```python
from build123d import *

# Parameters (mm, degrees)
EXTRUDE_1_DEPTH              = 5
HOLE_WIZARD_M4_1_D           = 4.3
HOLE_WIZARD_M4_1_CSINK_D     = 8.6
HOLE_WIZARD_M4_1_CSINK_ANGLE = 90
FILLET_1_R                   = 1


with BuildPart() as part:
    # 草图1 → 凸台-拉伸1 (new body)
    with BuildSketch(Plane(origin=(0, 0, 0), x_dir=(0, 0, -1), z_dir=(1, 0, 0))):
        Polygon((22, 18), (15.44969994, 18), (16.349099819, 8), (43.650900181, 8), (44.55030006, 18), (38, 18), align=None)
    extrude(amount=EXTRUDE_1_DEPTH)

    # M4 十字槽沉头木螺钉的锥形沉头孔1 (through all)
    with Locations(Plane.ZY):
        with Locations((-38, 13), (-22, 13)):
            CounterSinkHole(HOLE_WIZARD_M4_1_D / 2, HOLE_WIZARD_M4_1_CSINK_D / 2, counter_sink_angle=HOLE_WIZARD_M4_1_CSINK_ANGLE)

    # 圆角1
    # the kernel refuses this fillet: 1 mm, written as the material it takes off along each edge
    with BuildSketch(Plane(origin=(1, 9, -17.263196285), x_dir=(0, -0.08957840876297431, 0.9959797732301061), z_dir=(-1, 0, 0))) as fillet_1_piece_1_section:
        Polygon((0, 0), (FILLET_1_R, 0), (FILLET_1_R, -FILLET_1_R * 0.914096466321), (FILLET_1_R * 0.089578408763, -FILLET_1_R * 0.99597977323), align=None)
    fillet_1_piece_1 = extrude(amount=FILLET_1_R, mode=Mode.PRIVATE)
    fillet_1_piece_1 = fillet_1_piece_1 - Plane(origin=(1, 9, -17.263196285), x_dir=(0, 0.7380983703961737, -0.6746931121765753), z_dir=(-1, 0, 0)) * Sphere(FILLET_1_R, mode=Mode.PRIVATE)
    add(fillet_1_piece_1, mode=Mode.SUBTRACT)
    with BuildSketch(Plane(origin=(1, 9, -42.736803715), x_dir=(0, -1, 0), z_dir=(-1, 0, 0))) as fillet_1_piece_2_section:
        Polygon((0, 0), (FILLET_1_R, 0), (FILLET_1_R, -FILLET_1_R * 0.914096466321), (FILLET_1_R * 0.089578408763, -FILLET_1_R * 0.99597977323), align=None)
    fillet_1_piece_2 = extrude(amount=FILLET_1_R, mode=Mode.PRIVATE)
    fillet_1_piece_2 = fillet_1_piece_2 - Plane(origin=(1, 9, -42.736803715), x_dir=(0, 0.7380983703961737, 0.6746931121765753), z_dir=(-1, 0, 0)) * Sphere(FILLET_1_R, mode=Mode.PRIVATE)
    add(fillet_1_piece_2, mode=Mode.SUBTRACT)
    with BuildSketch(Plane(origin=(1, 17, -16.543676382), x_dir=(0, -0.08957840876297431, 0.9959797732301061), z_dir=(-1, 0, 0))) as fillet_1_piece_3_section:
        Polygon((0, 0), (FILLET_1_R, 0), (FILLET_1_R, FILLET_1_R * 1.09397644214), (-FILLET_1_R * 0.089578408763, FILLET_1_R * 0.99597977323), align=None)
    fillet_1_piece_3 = extrude(amount=FILLET_1_R, mode=Mode.PRIVATE)
    fillet_1_piece_3 = fillet_1_piece_3 - Plane(origin=(1, 17, -16.543676382), x_dir=(0, -0.6746931121765753, -0.7380983703961737), z_dir=(-1, 0, 0)) * Sphere(FILLET_1_R, mode=Mode.PRIVATE)
    add(fillet_1_piece_3, mode=Mode.SUBTRACT)
    with BuildSketch(Plane(origin=(1, 17, -43.456323618), x_dir=(0, -0.08957840876297431, -0.9959797732301061), z_dir=(-1, 0, 0))) as fillet_1_piece_4_section:
        Polygon((0, 0), (FILLET_1_R, 0), (FILLET_1_R, -FILLET_1_R * 1.09397644214), (-FILLET_1_R * 0.089578408763, -FILLET_1_R * 0.99597977323), align=None)
    fillet_1_piece_4 = extrude(amount=FILLET_1_R, mode=Mode.PRIVATE)
    fillet_1_piece_4 = fillet_1_piece_4 - Plane(origin=(1, 17, -43.456323618), x_dir=(0, -0.6746931121765753, 0.7380983703961737), z_dir=(-1, 0, 0)) * Sphere(FILLET_1_R, mode=Mode.PRIVATE)
    add(fillet_1_piece_4, mode=Mode.SUBTRACT)
    with BuildSketch(Plane(origin=(0, 8, -17.263196285), x_dir=(1, 0, 0), z_dir=(0, 0, -1))) as fillet_1_piece_5:
        with BuildLine():
            CenterArc((FILLET_1_R, -FILLET_1_R), FILLET_1_R, 90, 90)
            Line((0, -FILLET_1_R), (0, 0))
            Line((0, 0), (FILLET_1_R, 0))
        make_face()
    extrude(amount=25.47360743, mode=Mode.SUBTRACT)
    with BuildSketch(Plane(origin=(0, 16.910421591, -15.547696608), x_dir=(0, 0.08957840876297431, -0.9959797732301061), z_dir=(0, -0.9959797732301061, -0.08957840876297431))) as fillet_1_piece_6:
        with BuildLine():
            CenterArc((FILLET_1_R, FILLET_1_R), FILLET_1_R, 180, 90)
            Line((0, FILLET_1_R), (0, 0))
            Line((0, 0), (FILLET_1_R, 0))
        make_face()
    extrude(amount=8.032291634, mode=Mode.SUBTRACT)
    with BuildSketch(Plane(origin=(0, 18, -43.456323618), x_dir=(1, 0, 0), z_dir=(0, 0, 1))) as fillet_1_piece_7:
        with BuildLine():
            CenterArc((FILLET_1_R, -FILLET_1_R), FILLET_1_R, 90, 90)
            Line((0, -FILLET_1_R), (0, 0))
            Line((0, 0), (FILLET_1_R, 0))
        make_face()
    extrude(amount=26.912647237, mode=Mode.SUBTRACT)
    with BuildSketch(Plane(origin=(0, 8.910421591, -43.732783488), x_dir=(1, 0, 0), z_dir=(0, 0.9959797732301061, -0.08957840876297431))) as fillet_1_piece_8:
        with BuildLine():
            CenterArc((FILLET_1_R, -FILLET_1_R), FILLET_1_R, 90, 90)
            Line((0, -FILLET_1_R), (0, 0))
            Line((0, 0), (FILLET_1_R, 0))
        make_face()
    extrude(amount=8.032291634, mode=Mode.SUBTRACT)
    with BuildSketch(Plane(origin=(1, 8, -43.650900181), x_dir=(0, 0, 1), z_dir=(1, 0, 0))) as fillet_1_piece_9:
        with BuildLine():
            CenterArc((FILLET_1_R * 0.914096466321, -FILLET_1_R), FILLET_1_R, 90, 84.860646272)
            Line((-FILLET_1_R * 0.0818833069089, -FILLET_1_R * 0.910421591237), (0, 0))
            Line((0, 0), (FILLET_1_R * 0.914096466321, 0))
        make_face()
    extrude(amount=6.285241166, mode=Mode.SUBTRACT)
    with BuildSketch(Plane(origin=(1, 8, -16.349099819), x_dir=(0, 0, -1), z_dir=(1, 0, 0))) as fillet_1_piece_10:
        with BuildLine():
            CenterArc((FILLET_1_R * 0.914096466321, FILLET_1_R), FILLET_1_R, 185.139353728, 84.860646272)
            Line((-FILLET_1_R * 0.0818833069089, FILLET_1_R * 0.910421591237), (0, 0))
            Line((0, 0), (FILLET_1_R * 0.914096466321, 0))
        make_face()
    extrude(amount=6.285241166, mode=Mode.SUBTRACT)
    with BuildSketch(Plane(origin=(1, 18, -15.44969994), x_dir=(0, 0, -1), z_dir=(1, 0, 0))) as fillet_1_piece_11:
        with BuildLine():
            CenterArc((FILLET_1_R * 1.09397644214, -FILLET_1_R), FILLET_1_R, 90, 95.139353728)
            Line((FILLET_1_R * 0.0979966689112, -FILLET_1_R * 1.08957840876), (0, 0))
            Line((0, 0), (FILLET_1_R * 1.09397644214, 0))
        make_face()
    extrude(amount=6.734941105, mode=Mode.SUBTRACT)
    with BuildSketch(Plane(origin=(1, 18, -44.55030006), x_dir=(0, 0, 1), z_dir=(1, 0, 0))) as fillet_1_piece_12:
        with BuildLine():
            CenterArc((FILLET_1_R * 1.09397644214, FILLET_1_R), FILLET_1_R, 174.860646272, 95.139353728)
            Line((FILLET_1_R * 0.0979966689112, FILLET_1_R * 1.08957840876), (0, 0))
            Line((0, 0), (FILLET_1_R * 1.09397644214, 0))
        make_face()
    extrude(amount=6.734941105, mode=Mode.SUBTRACT)


solid = part.part
```
Check sheet for the modelled part. Datum: model origin and axes. Units: mm. Coordinates: 2 decimals unless noted, no trailing zeros. Order: outer loops, then holes, each group sorted by start corner. A loop starts at its lowest first (then second) coordinate and runs counter-clockwise, first axis right, second up. Notation, with made-up numbers: (16.5, -13.5) -> (65.5, -13.5) arc R14 ccw to (65.5, -2.5) -> close; hole circle Ø2 at (-5.75, 49). An arc over 180 degrees is marked (long way). Write item = value, one per line. Start each with the question number.
1) Cross-section at D-D (x = 0.3). Enter the section's corners in (y, z), then the cut area to 4 significant figures.
2) Go/stop test with flat-tipped pins: P1, Ø3, axis at x = 2, y = 13, coming from the -Z side; P2, Ø1, axis at x = 1, y = 11.5, coming from the -Z side. Record where each tip stops, or that it passes through.
3) Material ranges on L1, parallel to Z at x = 0.9, y = 12.5; L2, parallel to Z at x = 4.4, y = 13; L3, parallel to Y at x = 4.05, z = -22, recorded low to high.
4) Cross-section at B-B (z = -22). Enter the section's corners in (x, y), then the cut area to 3 significant figures.
5) Cross-section at A-A (x = 4.4). Enter the section's corners in (y, z).
6) Mould release check, pull along Z, two halves, no side actions. Record for faces 1 (the cylindrical face through (2.97, 17.68, -15.81)), 2 (the cylindrical face through (3.59, 11.09, -22.99)), 3 (the flat face through (3, 8, -30)): +Z half, -Z half, draft (parallel to the pull), parting line (faces both ways), or undercut.
7) Cross-section at C-C (y = 13). State how many separate pieces and enclosed holes the cut face has, then the cut area to 3 significant figures.
Ans:
q1.outline = (8.29, -42.74) arc R0.71 ccw to (8.94, -43.45) -> (16.94, -44.17) arc R0.71 ccw to (17.71, -43.46) -> (17.71, -16.54) arc R0.71 ccw to (16.94, -15.83) -> (8.94, -16.55) arc R0.71 ccw to (8.29, -17.26) -> close; hole circle Ø8 at (13, -38); hole circle Ø8 at (13, -22)
q1.area = 159.5 mm²
q2.P1 = -44.24
q2.P2 = -44.01
q3.L1 = -44.05 to -41.36, -34.64 to -25.36, -18.64 to -15.95
q3.L2 = -44.1 to -40.15, -35.85 to -24.15, -19.85 to -15.9
q3.L3 = 8 to 10.85, 15.15 to 18
q4.outline = (0.04, 8.74) arc R1 ccw to (1, 8) -> (5, 8) -> (5, 10.85) -> (2.15, 10.85) -> close; (0.04, 17.26) -> (2.15, 15.15) -> (5, 15.15) -> (5, 18) -> (1, 18) arc R1 ccw to start
q4.area = 23.5 mm²
q5.outline = (8, -42.74) arc R1 ccw to (8.91, -43.73) -> (16.91, -44.45) arc R1 ccw to (18, -43.46) -> (18, -16.54) arc R1 ccw to (16.91, -15.55) -> (8.91, -16.27) arc R1 ccw to (8, -17.26) -> close; hole circle Ø4.3 at (13, -38); hole circle Ø4.3 at (13, -22)
q6.face_1 = +Z half
q6.face_2 = undercut
q6.face_3 = draft
q7.separate_pieces = 3
q7.enclosed_holes = 0
q7.area = 88.3 mm²
